Could you check a few things on this model? Use its own coordinates, in mm. Face numbers are marked on the shaded views. A direction names the side the tool comes from. Give positions to 0.01 mm unless a question says otherwise; leave off trailing zeros. Write each loop counter-clockwise with the first axis right and the second up, starting at its lowest first coordinate (ties: lowest second). Pieces come first, ordered by that corner, then holes. Notation, with made-up numbers: (82, 1.25) -> (132, 1.25) arc R32 cw to (132, 33.25) -> close; hole circle Ø11 at (25, -1.5). An arc over 180 degrees is marked (long way). One line per question, with ' | ' between items.
from build123d import *

# Parameters (mm, degrees)
SKETCH1_R           = 5
SKETCH1_R_2         = 14.85
BOSS_EXTRUDE1_DEPTH = 18.61
SKETCH3_R           = 37.94
SKETCH3_R_2         = 24
CUT_EXTRUDE1_DEPTH  = 6.8
SKETCH4_R           = 14.35
BOSS_EXTRUDE2_DEPTH = 50.95
SKETCH5_R           = 5
CUT_EXTRUDE2_DEPTH  = 27.24
FILLET1_R           = 4


with BuildPart() as part:
    # Sketch1 → Boss-Extrude1 (new body)
    with BuildSketch(Plane.XY):
        with BuildLine():
            Line((44.744350737, 34.662704412), (44.744350737, 0.617322885))
            ThreePointArc((44.744350737, 0.617322885), (43.097385261, -10.288147364), (38.303391852, -20.220891388))
            Line((38.303391852, -20.220891388), (14.7812281, -54.635842593))
            ThreePointArc((14.7812281, -54.635842593), (0, -56.6), (-14.7812281, -54.635842593))
            Line((-14.7812281, -54.635842593), (-38.299041115, -20.22725689))
            ThreePointArc((-38.299041115, -20.22725689), (-43.093034524, -10.294512867), (-44.74, 0.610957382))
            Line((-44.74, 0.610957382), (-44.74, 34.668319832))
            ThreePointArc((-44.74, 34.668319832), (0.003551826, 56.599999889), (44.744350737, 34.662704412))
        make_face()
        with Locations((0, 44.95)):
            Circle(SKETCH1_R, mode=Mode.SUBTRACT)
        Circle(SKETCH1_R_2, mode=Mode.SUBTRACT)
    extrude(amount=-BOSS_EXTRUDE1_DEPTH)

    # Sketch3 → Cut-Extrude1 (cut)
    with BuildSketch(Plane.XY):
        Circle(SKETCH3_R)
        Circle(SKETCH3_R_2, mode=Mode.SUBTRACT)
    extrude(amount=-CUT_EXTRUDE1_DEPTH, mode=Mode.SUBTRACT)

    # Sketch4 → Boss-Extrude2 (add)
    with BuildSketch(Plane.XY.offset(-6.8)):
        with Locations((0, -32.4)):
            Circle(SKETCH4_R)
    extrude(amount=-BOSS_EXTRUDE2_DEPTH)

    # Sketch5 → Cut-Extrude2 (cut)
    with BuildSketch(Plane.XY.offset(-6.8)):
        with Locations((0, -32.4)):
            Circle(SKETCH5_R)
    extrude(amount=-CUT_EXTRUDE2_DEPTH, mode=Mode.SUBTRACT)

    # Fillet1
    fillet1_edges = [part.edges().sort_by_distance(p)[0] for p in [
        (-24, 0, -6.8),
    ]]
    fillet(fillet1_edges, radius=FILLET1_R)


solid = part.part
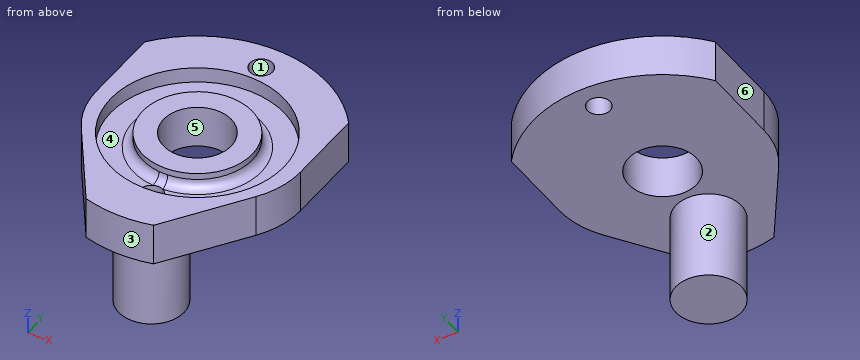
Q1. If we mould it in two halves opening along X, with no side actions, what happens to the marked faces 3, 4, 5 and 6? For each: +X half, -X half, draft (parallel to the pull), parting line (faces both ways), or undercut.
Answer below:
face 3: parting line | face 4: undercut | face 5: undercut | face 6: -X half
Q2. Imagine slicing it at D-D on z = -43. Please give me the cut outline in (x, y).
Answer below:
outline: circle Ø28.7 at (0, -32.4)
Q3. On a 3-axis mill with a long thin cutter (end or side, diameter ignored), from which of +Z, -Z, +X, -X, +Y, -Y can I reach the whole of each face in a straight line? I mean the marked faces 1 and 2. Say none if no direction works.
Answer below:
face 1: +Z, -Z | face 2: -Z
Q4. Will these pins go through, and if not, where does the flat tip stop? pin 1 (6 mm diameter, centred on x = 21.5, z = -10.5, fed in from -Y); pin 2 (10 mm diameter, centred on x = -1, z = -33.5, fed in from +Y); pin 3 (1.5 mm diameter, centred on x = 10, z = -43.5, fed in from +Y).
Answer below:
pin 1: stops at y = -49.19 | pin 2: stops at y = -18.05 | pin 3: stops at y = -21.43
Q5. If I drill on line 1 along Y through (x, z) = (0, -3) (3 decimals); line 2 along Y through (x, z) = (0, -5.25); line 3 along Y through (x, z) = (0, -16), over which ranges is the centre line in solid material (lowest first)?
Answer below:
line 1: y = -56.6 to -37.94, -24.003 to -14.85, 14.85 to 24.005, 37.94 to 39.95, 49.95 to 56.6 | line 2: y = -56.6 to -37.94, -24.8 to -14.85, 14.85 to 24.84, 37.94 to 39.95, 49.95 to 56.6 | line 3: y = -56.6 to -37.4, -27.4 to -14.85, 14.85 to 39.95, 49.95 to 56.6
Q6. Imagine slicing it at B-B on x = 0. Count the separate pieces of the cut face and the enclosed holes in it, and give its area (3 significant figures).
Answer below:
separate pieces: 3 | enclosed holes: 0 | area: 2,040 mm^2
Q7. Imagine slicing it at A-A on z = -12. Please give me the cut outline in (x, y), and give its area (3 significant figures).
Answer below:
outline: (-44.74, 0.61) arc R36.93 ccw to (-38.3, -20.23) -> (-14.78, -54.64) arc R56.6 ccw to (14.78, -54.64) -> (38.3, -20.22) arc R36.93 ccw to (44.74, 0.62) -> (44.74, 34.66) arc R56.6 ccw to (-44.74, 34.67) -> close; hole circle Ø29.7 at (0, 0); hole circle Ø10 at (0, -32.4); hole circle Ø10 at (0, 44.95) | area: 7,210 mm^2
Q8. Imagine slicing it at C-C on y = 44.95. Please give me the cut outline in (x, z), and give its area (3 significant figures).
Answer below:
outline: (-34.4, -18.61) -> (-5, -18.61) -> (-5, 0) -> (-34.4, 0) -> close; (5, -18.61) -> (34.4, -18.61) -> (34.4, 0) -> (5, 0) -> close | area: 1,090 mm^2
